Can you work these out from the model? Positions are in its coordinate system, mm. A direction names the side the tool comes from. Round coordinates to 2 decimals unless told otherwise and drop trailing zeros. Loops run counter-clockwise (first coordinate to the right, second up) from the corner with the lowest first, then second, coordinate; pieces in that order, holes last. Notation, with made-up numbers: (-39, -15) -> (-4, -15) arc R16 cw to (-4, 1) -> close; hole circle Ø6 at (-36.5, 60). An arc over 180 degrees is marked (long way). Answer as a JSON object with one key per item and string values.
```python
from build123d import *

# Parameters (mm, degrees)
SKETCH_1_R      = 3.5775
SKETCH_1_R_2    = 0.19875
EXTRUDE_2_DEPTH = 0.159
EXTRUDE_START   = 0.3975
SKETCH_1_6_R    = 0.19875
EXTRUDE_3_DEPTH = 0.3975


with BuildPart() as part:
    # Sketch 1 → Extrude 2 (new body)
    # profile 1 of 3: a face of its own
    with BuildSketch(Plane.XY):
        Circle(SKETCH_1_R)
        with Locations((-3.18, 0)):
            Circle(SKETCH_1_R_2, mode=Mode.SUBTRACT)
        with BuildLine():
            ThreePointArc((-1.985091803, -1.949799165), (2.7825, 0), (-1.985091803, 1.949799165))
            ThreePointArc((-1.985091803, 1.949799165), (-1.317199128, 0), (-1.985091803, -1.949799165))
        make_face(mode=Mode.SUBTRACT)
    # profile 2 of 3: a face of its own
    with BuildSketch(Plane.XY):
        with BuildLine():
            ThreePointArc((-1.985091803, -1.949799165), (-1.317199128, 0), (-1.985091803, 1.949799165))
            ThreePointArc((-1.985091803, 1.949799165), (2.7825, 0), (-1.985091803, -1.949799165))
        make_face()
        Circle(SKETCH_1_R_2, mode=Mode.SUBTRACT)
    # profile 3 of 3: a face of its own
    with BuildSketch(Plane.XY):
        with Locations((-3.18, 0)):
            Circle(SKETCH_1_R_2)
    extrude(amount=-EXTRUDE_2_DEPTH)

    # Sketch 1_6 → Extrude 3 (add)
    # profile 1 of 2: a face of its own
    with BuildSketch(Plane.XY.offset(EXTRUDE_START)):
        with BuildLine():
            ThreePointArc((-1.985091803, -1.949799165), (-1.317199128, 0), (-1.985091803, 1.949799165))
            ThreePointArc((-1.985091803, 1.949799165), (2.7825, 0), (-1.985091803, -1.949799165))
        make_face()
        Circle(SKETCH_1_6_R, mode=Mode.SUBTRACT)
    # profile 2 of 2: a face of its own
    with BuildSketch(Plane.XY.offset(EXTRUDE_START)):
        with Locations((-3.18, 0)):
            Circle(SKETCH_1_6_R)
    extrude(amount=-EXTRUDE_3_DEPTH)


solid = part.part
```
Q1. If I drill on L1, parallel to Y at x = 0, z = 0.2; L2, parallel to Z at x = 2, y = -2; L3, parallel to X at y = -0.25, z = 0.1, over which ranges is the centre line in solid material (lowest first)? Write a range as [from, to].
Determined:
{"L1": "[-2.78, -0.2], [0.2, 2.78]", "L2": "[-0.16, 0]", "L3": "[-1.33, 2.77]"}
Q2. I want a section at C-C, the plane z = 0.2. Write out the boundary of the cut face in (x, y) (1 decimal), then the cut area to 3 significant figures.
Determined:
{"outline": "circle Ø0.4 at (-3.2, 0); (-2, -1.9) arc R2.8 ccw (long way) to (-2, 1.9) arc R3.2 cw to start; hole circle Ø0.4 at (0, 0)", "area": "20.4 mm²"}
Q3. I want a section at A-A, the plane x = 0. Write out the boundary of the cut face in (y, z).
Determined:
{"outline": "(-3.58, -0.16) -> (-0.2, -0.16) -> (-0.2, 0.4) -> (-2.78, 0.4) -> (-2.78, 0) -> (-3.58, 0) -> close; (0.2, -0.16) -> (3.58, -0.16) -> (3.58, 0) -> (2.78, 0) -> (2.78, 0.4) -> (0.2, 0.4) -> close"}
Q4. I want a section at B-B, the plane y = 0. Write out the boundary of the cut face in (x, z).
Determined:
{"outline": "(-3.58, -0.16) -> (-0.2, -0.16) -> (-0.2, 0.4) -> (-1.32, 0.4) -> (-1.32, 0) -> (-2.98, 0) -> (-2.98, 0.4) -> (-3.38, 0.4) -> (-3.38, 0) -> (-3.58, 0) -> close; (0.2, -0.16) -> (3.58, -0.16) -> (3.58, 0) -> (2.78, 0) -> (2.78, 0.4) -> (0.2, 0.4) -> close"}
Q5. On a 3-axis mill with a long thin cutter (end or side, diameter ignored), from which of +Z, -Z, +X, -X, +Y, -Y can I reach the whole of each face in a straight line? I mean faces 1 (the flat face through (0.4, 0, 0.398)), 2 (the cylindrical face through (2.78, 0.09, 0.2)). Say none if no direction works.
Determined:
{"face 1": "+Z, +X, -X, +Y, -Y", "face 2": "+Z"}
Q6. I want a section at D-D, the plane x = -1.5. Write out the boundary of the cut face in (y, z), then the cut area to 3 significant figures.
Determined:
{"outline": "(-3.25, -0.16) -> (3.25, -0.16) -> (3.25, 0) -> (2.34, 0) -> (2.34, 0.4) -> (1.06, 0.4) -> (1.06, 0) -> (-1.06, 0) -> (-1.06, 0.4) -> (-2.34, 0.4) -> (-2.34, 0) -> (-3.25, 0) -> close", "area": "2.05 mm²"}
